from build123d import *

# Parameters (mm, degrees)
SKETCH_W        = 40
SKETCH_H        = 93
PAD_DEPTH       = 4.5
SKETCH001_R     = 2.2
POCKET_DEPTH    = 5
FILLET_R        = 3
SKETCH002_R     = 3.1
POCKET001_DEPTH = 5
SKETCH003_W     = 15
SKETCH003_H     = 8.1
PAD001_DEPTH    = 1.8


with BuildPart() as part:
    # Sketch → Pad (new body)
    with BuildSketch(Plane.XY):
        with Locations((0, 16.5)):
            Rectangle(SKETCH_W, SKETCH_H)
    extrude(amount=PAD_DEPTH)

    # Sketch001 (on Face6 of Pad) → Pocket (cut)
    with BuildSketch(Plane.XY.offset(4.5)):
        with Locations((-15, 58.3)):
            Circle(SKETCH001_R)
        with Locations((15, 58.3)):
            Circle(SKETCH001_R)
        with Locations((0, 58.3)):
            Circle(SKETCH001_R)
        with Locations((-15, 4)):
            Circle(SKETCH001_R)
        with Locations((0, 4)):
            Circle(SKETCH001_R)
        with Locations((15, 4)):
            Circle(SKETCH001_R)
    extrude(amount=-POCKET_DEPTH, mode=Mode.SUBTRACT)

    # Fillet
    fillet_edges = [part.edges().sort_by_distance(p)[0] for p in [
        (20, 63, 2.25),
        (-20, 63, 2.25),
    ]]
    fillet(fillet_edges, radius=FILLET_R)

    # Sketch002 (on Face5 of Fillet) → Pocket001 (cut)
    with BuildSketch(Plane.XY.offset(4.5)):
        with Locations((0, -15)):
            Circle(SKETCH002_R)
    extrude(amount=-POCKET001_DEPTH, mode=Mode.SUBTRACT)

    # Sketch003 (on Face2 of Pocket001) → Pad001 (join)
    with BuildSketch(Plane(origin=(0, 0, 0), x_dir=(1, 0, 0), z_dir=(0, 0, -1))):
        with Locations((-12.5, 15)):
            Rectangle(SKETCH003_W, SKETCH003_H)
        with Locations((12.5, 15)):
            Rectangle(SKETCH003_W, SKETCH003_H)
    extrude(amount=PAD001_DEPTH)


solid = part.part
CAD build for the part. Positions are in the model's coordinates, mm. A direction names the side the tool comes from. Round coordinates to 2 decimals unless told otherwise and drop trailing zeros. Order: outer loops, then holes, each group sorted by start corner. A loop starts at its lowest first (then second) coordinate and runs counter-clockwise, first axis right, second up. Notation, with made-up numbers: M -9,27 L 8,27 A15 ccw 8,37 Z; hole C -22,15 d4. An arc over 180 degrees is marked long. Use one line per item in the form item = value.
Q1. Two-plate mould, pull along X, no slides. Class faces 1 (the cylindrical face through (-19.14, 62.1, 2.28)), 2 (the flat face through (12, -15, -1.8)), 3 (the cylindrical face through (17.032, 3.157, 2.282)): +X half, -X half, draft (parallel to the pull), parting line (faces both ways), or undercut.
Recorded:
face_1 = -X half
face_2 = draft
face_3 = undercut
Q2. Which spindle directions (+Z, -Z, +X, -X, +Y, -Y) get a long thin tool onto all of the face, cutting with end or side? Do faces 4 (the flat face through (12, -19.05, -1)), 5 (the flat face through (12, -10.95, -1)), 6 (the flat face through (5, -15, -1)). Say none if no direction does.
Recorded:
face_4 = -Z, +X, -X, -Y
face_5 = -Z, +X, -X, +Y
face_6 = -Z, +Y, -Y
Q3. Saw through at B-B on y = 58.3. Give the cut face in (x, z), then the cut area to 3 significant figures.
Recorded:
outline = M -20,0 L -17.2,0 L -17.2,4.5 L -20,4.5 Z; M -12.8,0 L -2.2,0 L -2.2,4.5 L -12.8,4.5 Z; M 2.2,0 L 12.8,0 L 12.8,4.5 L 2.2,4.5 Z; M 17.2,0 L 20,0 L 20,4.5 L 17.2,4.5 Z
area = 121 mm^2
Q4. Flat gauge pins, fed straight in: P1, Ø0.9, axis at x = 14.5, z = -1, coming from the -Y side; P2, Ø20, axis at x = 7, y = 2.5, coming from the -Z side; P3, Ø0.5, axis at x = -15.5, z = -1, coming from the +Y side; P4, Ø5.5, axis at x = 0, y = 58.3, coming from the +Z side. Where does each tip first touch, or does it go through?
Recorded:
P1 = -19.05
P2 = 0
P3 = -10.95
P4 = 4.5
Q5. Saw through at D-D on x = -15. Give the cut face in (y, z).
Recorded:
outline = M -30,0 L -19.05,0 L -19.05,-1.8 L -10.95,-1.8 L -10.95,0 L 1.8,0 L 1.8,4.5 L -30,4.5 Z; M 6.2,0 L 56.1,0 L 56.1,4.5 L 6.2,4.5 Z; M 60.5,0 L 63,0 L 63,4.5 L 60.5,4.5 Z
Q6. Probe L1, parallel to Y at x = -15, z = 1.9; L2, parallel to X at y = 3, z = 0.5; L3, parallel to Y at x = -14, z = 2.5. List the from-to ranges inside material, lowest first.
Recorded:
L1 = -30 to 1.8, 6.2 to 56.1, 60.5 to 63
L2 = -20 to -16.96, -13.04 to -1.96, 1.96 to 13.04, 16.96 to 20
L3 = -30 to 2.04, 5.96 to 56.34, 60.26 to 63
Q7. Saw through at C-C on y = -15. Give the cut face in (x, z).
Recorded:
outline = M -20,-1.8 L -5,-1.8 L -5,0 L -3.1,0 L -3.1,4.5 L -20,4.5 Z; M 3.1,0 L 5,0 L 5,-1.8 L 20,-1.8 L 20,4.5 L 3.1,4.5 Z
Q8. Saw through at A-A on x = 0. Give the cut face in (y, z), then the cut area to 3 significant figures.
Recorded:
outline = M -30,0 L -18.1,0 L -18.1,4.5 L -30,4.5 Z; M -11.9,0 L 1.8,0 L 1.8,4.5 L -11.9,4.5 Z; M 6.2,0 L 56.1,0 L 56.1,4.5 L 6.2,4.5 Z; M 60.5,0 L 63,0 L 63,4.5 L 60.5,4.5 Z
area = 351 mm^2
